from build123d import *

# Parameters (mm, degrees)
F1_DEPTH = 2.5
F2_R     = 0.85
F3_DEPTH = 12.5


with BuildPart() as f1:
    # F0 (on Top) → F1 (new body)
    with BuildSketch(Plane.XY):
        with BuildLine():
            Line((13.081475452, -13.081475452), (1.0606601718, -1.0606601718))
            ThreePointArc((1.0606601718, -1.0606601718), (0, -0.6213203436), (-1.0606601718, -1.0606601718))
            Line((-1.0606601718, -1.0606601718), (-13.081475452, -13.081475452))
            ThreePointArc((-13.081475452, -13.081475452), (-13.5208152802, -14.1421356237), (-13.081475452, -15.2027957955))
            Line((-13.081475452, -15.2027957955), (-1.0606601718, -27.2236110757))
            ThreePointArc((-1.0606601718, -27.2236110757), (0, -27.6629509039), (1.0606601718, -27.2236110757))
            Line((1.0606601718, -27.2236110757), (13.081475452, -15.2027957955))
            ThreePointArc((13.081475452, -15.2027957955), (13.5208152802, -14.1421356237), (13.081475452, -13.081475452))
        make_face()
        with BuildLine():
            Line((-4.0470226145, -10.1208059821), (-5.0821788645, -10.1208059821))
            Line((-5.0821788645, -10.1208059821), (-5.0821788645, -12.1824379265))
            Line((-5.0821788645, -12.1824379265), (-5.6583507395, -12.1824379265))
            Line((-5.6583507395, -12.1824379265), (-5.6583507395, -7.2247556349))
            Line((-5.6583507395, -7.2247556349), (-4.2987587256, -7.2247556349))
            add(Edge.make_bspline(
                [(-4.2987587256, -7.2247556349), (-3.3862153229, -7.2247556349), (-2.9505599409, -7.574147996)],
                knots=[0, 0, 0, 1, 1, 1], degree=2))
            add(Edge.make_bspline(
                [(-2.9505599409, -7.574147996), (-2.514904559, -7.9235403571), (-2.514904559, -8.6255802876)],
                knots=[0, 0, 0, 1, 1, 1], degree=2))
            add(Edge.make_bspline(
                [(-2.514904559, -8.6255802876), (-2.514904559, -9.6086532043), (-3.5120833784, -9.9547903571)],
                knots=[0, 0, 0, 1, 1, 1], degree=2))
            Line((-3.5120833784, -9.9547903571), (-2.1655121979, -12.1824379265))
            Line((-2.1655121979, -12.1824379265), (-2.846935809, -12.1824379265))
            Line((-2.846935809, -12.1824379265), (-4.0470226145, -10.1208059821))
        make_face(mode=Mode.SUBTRACT)
        with BuildLine():
            Line((-8.1334756687, -14.8039748892), (-8.1334756687, -13.4802963582))
            Line((-8.1334756687, -13.4802963582), (-0.6236797201, -13.4802963582))
            Line((-0.6236797201, -13.4802963582), (-0.6236797201, -6.9198086858))
            ThreePointArc((-0.6236797201, -6.9198086858), (-0.9032194318, -6.4583786209), (-0.9135835525, -5.9189782686))
            ThreePointArc((-0.9135835525, -5.9189782686), (0.0168397474, -5.0141534426), (0.9868078824, -5.876451129))
            ThreePointArc((0.9868078824, -5.876451129), (0.9900106564, -6.4384308628), (0.6999988109, -6.9198086858))
            Line((0.6999988109, -6.9198086858), (0.6999988109, -13.4802963582))
            Line((0.6999988109, -13.4802963582), (8.1334756687, -13.4802963582))
            ThreePointArc((8.1334756687, -13.4802963582), (8.5949057336, -13.2007566465), (9.134306086, -13.1903925258))
            ThreePointArc((9.134306086, -13.1903925258), (10.0391309119, -14.1208158258), (9.1768332255, -15.0907839607))
            ThreePointArc((9.1768332255, -15.0907839607), (8.6148534917, -15.0939867347), (8.1334756687, -14.8039748892))
            Line((8.1334756687, -14.8039748892), (0.6999988109, -14.8039748892))
            Line((0.6999988109, -14.8039748892), (0.6999988109, -23.1867600232))
            Line((0.6999988109, -23.1867600232), (-0.6236797201, -23.1867600232))
            Line((-0.6236797201, -23.1867600232), (-0.6236797201, -14.8039748892))
            Line((-0.6236797201, -14.8039748892), (-8.1334756687, -14.8039748892))
        make_face(mode=Mode.SUBTRACT)
        with BuildLine():
            add(Edge.make_bspline(
                [(3.0161563763, -12.5007560808), (2.690635543, -12.8550312544), (2.0797414457, -12.8550312544)],
                knots=[0, 0, 0, 1, 1, 1], degree=2))
            add(Edge.make_bspline(
                [(2.0797414457, -12.8550312544), (1.7618160985, -12.8550312544), (1.5784393624, -12.7638854211)],
                knots=[0, 0, 0, 1, 1, 1], degree=2))
            Line((1.5784393624, -12.7638854211), (1.5784393624, -12.2723489627))
            add(Edge.make_bspline(
                [(1.5784393624, -12.2723489627), (1.8193247791, -12.3396232683), (2.0797414457, -12.3396232683)],
                knots=[0, 0, 0, 1, 1, 1], degree=2))
            add(Edge.make_bspline(
                [(2.0797414457, -12.3396232683), (2.4161129735, -12.3396232683), (2.5908091541, -12.1361727474)],
                knots=[0, 0, 0, 1, 1, 1], degree=2))
            add(Edge.make_bspline(
                [(2.5908091541, -12.1361727474), (2.7655053346, -11.9327222266), (2.7655053346, -11.5496927127)],
                knots=[0, 0, 0, 1, 1, 1], degree=2))
            Line((2.7655053346, -11.5496927127), (2.7655053346, -6.5920104211))
            Line((2.7655053346, -6.5920104211), (3.3416772096, -6.5920104211))
            Line((3.3416772096, -6.5920104211), (3.3416772096, -11.5019496572))
            add(Edge.make_bspline(
                [(3.3416772096, -11.5019496572), (3.3416772096, -12.1464809072), (3.0161563763, -12.5007560808)],
                knots=[0, 0, 0, 1, 1, 1], degree=2))
        make_face(mode=Mode.SUBTRACT)
    extrude(amount=F1_DEPTH)

    # F2 (on Right) → F3 (cut, symmetric)
    with BuildSketch(Plane.YZ):
        with Locations((-2.4908210296, 1.292226194)):
            Circle(F2_R)
    extrude(amount=F3_DEPTH, both=True, mode=Mode.SUBTRACT)


solid = f1.part
Work out the finished part from the listing and answer in its coordinate system (mm). A direction names the side the tool comes from. Round coordinates to 2 decimals unless told otherwise and drop trailing zeros. Write each loop counter-clockwise with the first axis right and the second up, starting at its lowest first coordinate (ties: lowest second). Pieces come first, ordered by that corner, then holes.
1) A cutting plane is placed at B-B (y = -2.25). Give the vertices of the cut face in (x, z), plus the area to 3 significant figures.
2) A tool of negligible diameter and unlimited length cuts with its end or side. For faces 4 (the flat face through (-0.624, -10, 1)), 5 (the flat face through (6.987, -21.297, 1.232)), from which of +Z, -Z, +X, -X, +Y, -Y can it reach the whole face along a straight path? Write none if from no direction.
3) Given pin 1 Ø1.2 at (y, z) = (-20, 1) entering from -X; pin 2 Ø1.5 at (y, z) = (-6.5, 2) entering from -X; pin 3 Ø0.8 at (y, z) = (-9, 1.5) entering from +X, each flat-ended and moving along its own axis, determine where each tip first touches the part or whether it passes through.
4) A cutting plane is placed at A-A (x = 0). Give the vertices of the cut face in (y, z).
5) A cutting plane is placed at C-C (x = 4.5). Give the vertices of the cut face in (y, z), plus the area to 3 significant figures.
6) A cutting plane is placed at D-D (z = 0.75). Give the number of separate pieces and of enclosed holes in the cut face, plus the area to 3 significant figures.
7) The mould has two halves that part along X. Classify faces 1 (the cylindrical face through (13.52, -14.16, 1.23)), 2 (the cylindrical face through (-13.52, -14.13, 1.23)), 3 (the flat face through (-2.85, -11.05, 1.23)): pulls with the +X half, pulls with the -X half, needs draft (parallel to the pull), parting line crosses it, or undercut.
8) Straight lines are drawn through the part: line 1 (X direction, y = -10, z = 0.35); line 2 (X direction, y = -9, z = 0.5); line 3 (Y direction, x = -3.75, z = 2.2). For each, find the intervals that lie inside material, in ascending order.
Completed:
1. outline: (-2.25, 0) - (2.25, 0) - (2.25, 0.48) - (-2.25, 0.48) - close; (-2.25, 2.11) - (2.25, 2.11) - (2.25, 2.5) - (-2.25, 2.5) - close
1. area: 3.91 mm2
2. face 4: +Z, -Z
2. face 5: +Z, -Z, +X, -Y
3. pin 1: stops at x = -8.88
3. pin 2: stops at x = -7.25
3. pin 3: stops at x = 9.4
4. outline: (-27.66, 0) - (-23.19, 0) - (-23.19, 2.5) - (-27.66, 2.5) - close; (-5.01, 0) - (-0.62, 0) - (-0.62, 2.5) - (-5.01, 2.5) - close; hole circle Ø1.7 at (-2.49, 1.29)
5. outline: (-23.78, 0) - (-14.8, 0) - (-14.8, 2.5) - (-23.78, 2.5) - close; (-13.48, 0) - (-4.5, 0) - (-4.5, 2.5) - (-13.48, 2.5) - close
5. area: 44.9 mm2
6. separate pieces: 2
6. enclosed holes: 3
6. area: 329 mm2
7. face 1: pulls with the +X half
7. face 2: pulls with the -X half
7. face 3: undercut
8. line 1: x = -10 to -5.66, -3.48 to -0.62, 0.7 to 2.77, 3.34 to 10
8. line 2: x = -9 to -5.66, -2.56 to -0.62, 0.7 to 2.77, 3.34 to 9
8. line 3: y = -24.53 to -14.8, -13.48 to -10.63, -7.26 to -3.75
